Read the model definition and answer for the solid it produces. Units are mm, in the model's axes. Give positions to 0.01 mm unless a question says otherwise; leave off trailing zeros. Write each loop counter-clockwise with the first axis right and the second up, starting at its lowest first coordinate (ties: lowest second). Pieces come first, ordered by that corner, then holes. Notation, with made-up numbers: (31.5, 66) -> (82.5, 66) arc R17 cw to (82.5, 94) -> close; hole circle Ø9 at (-18.75, 28). An arc over 180 degrees is marked (long way). Write item = value, one per line.
from build123d import *

# Parameters (mm, degrees)
SKETCH1_R           = 74.676
BOSS_EXTRUDE1_DEPTH = 3.175
SKETCH2_R           = 7
CUT_EXTRUDE1_DEPTH  = 106.655527906
SKETCH3_R           = 2.25
CUT_EXTRUDE2_DEPTH  = 106.655527906
SKETCH4_R           = 3.175
CUT_EXTRUDE3_DEPTH  = 106.655527906
CUT_EXTRUDE5_REACH  = 107.656
SKETCH6_R           = 6.35


with BuildPart() as part:
    # Sketch1 → Boss-Extrude1 (new body)
    with BuildSketch(Plane(origin=(0, 0, 0), x_dir=(1, 0, 0), z_dir=(0, 1, 0))):
        with Locations(Location((0, 0, 0), (0, 0, 270))):
            Circle(SKETCH1_R)
    extrude(amount=BOSS_EXTRUDE1_DEPTH)

    # Sketch2 → Cut-Extrude1 (cut, through all)
    with BuildSketch(Plane(origin=(0, 3.175, 0), x_dir=(1, 0, 0), z_dir=(0, 1, 0))):
        with Locations(Location((0, 0, 0), (0, 0, 270))):
            Circle(SKETCH2_R)
    extrude(amount=-CUT_EXTRUDE1_DEPTH, mode=Mode.SUBTRACT)

    # Sketch3 → Cut-Extrude2 (cut, through all)
    with BuildSketch(Plane(origin=(0, 3.175, 0), x_dir=(1, 0, 0), z_dir=(0, 1, 0))):
        with Locations(Location((11.314, 0, 0), (0, 0, 270))):
            Circle(SKETCH3_R)
        with Locations(Location((0, -11.314, 0), (0, 0, 270))):
            Circle(SKETCH3_R)
        with Locations(Location((-11.314, 0, 0), (0, 0, 270))):
            Circle(SKETCH3_R)
        with Locations(Location((0, 11.314, 0), (0, 0, 270))):
            Circle(SKETCH3_R)
    extrude(amount=-CUT_EXTRUDE2_DEPTH, mode=Mode.SUBTRACT)

    # Sketch4 → Cut-Extrude3 (cut, through all)
    with BuildSketch(Plane(origin=(0, 3.175, 0), x_dir=(1, 0, 0), z_dir=(0, 1, 0))):
        with Locations(Location((50.8, 0, 0), (0, 0, 270))):
            Circle(SKETCH4_R)
        with Locations(Location((-50.8, 0, 0), (0, 0, 270))):
            Circle(SKETCH4_R)
    extrude(amount=-CUT_EXTRUDE3_DEPTH, mode=Mode.SUBTRACT)

    # Sketch6 → Cut-Extrude5 (cut, up to next)
    with BuildSketch(Plane(origin=(0, 3.175, 0), x_dir=(1, 0, 0), z_dir=(0, 1, 0)), mode=Mode.PRIVATE) as cut_extrude5_sk1:
        with Locations(Location((0, 41.73382544, 0), (0, 0, 270))):
            Circle(SKETCH6_R)
    cut_extrude5_tool1 = extrude(cut_extrude5_sk1.sketch, amount=-CUT_EXTRUDE5_REACH, mode=Mode.PRIVATE) & part.part
    add(cut_extrude5_tool1.solids().sort_by_distance((0, 3.175, -41.733825))[0], mode=Mode.SUBTRACT)


solid = part.part
(1) Given P1, Ø1.5, axis at y = 0.5, z = 35, coming from the -X side; P2, Ø1, axis at y = 2.5, z = -46.5, coming from the -X side, each flat-ended and moving along its own axis, determine where each tip first touches the part or whether it passes through.
Checks:
P1 = -66.36
P2 = -58.83
(2) For a pull along Z with two mould halves and no side action, classify faces 1 (the cylindrical face through (22.431, 1.565, 71.228)), 2 (the cylindrical face through (-6.834, 1.61, -1.517)), 3 (the flat face through (-16, 3.175, -1)) as released by +Z, released by -Z, zero draft, split by the parting line, or undercut.
Checks:
face_1 = split by the parting line
face_2 = undercut
face_3 = zero draft
(3) The part is cut by section B-B on z = -45. Determine the outline of the cut face in (x, y) (1 decimal), plus the area to 3 significant figures.
Checks:
outline = (-59.6, 0) -> (-5.4, 0) -> (-5.4, 3.2) -> (-59.6, 3.2) -> close; (5.4, 0) -> (59.6, 0) -> (59.6, 3.2) -> (5.4, 3.2) -> close
area = 344 mm²
(4) The part is cut by section C-C on x = 50.8. Determine the outline of the cut face in (y, z) (1 decimal), plus the area to 3 significant figures.
Checks:
outline = (0, -54.7) -> (3.2, -54.7) -> (3.2, -3.2) -> (0, -3.2) -> close; (0, 3.2) -> (3.2, 3.2) -> (3.2, 54.7) -> (0, 54.7) -> close
area = 327 mm²
(5) Consider L1, parallel to X at y = 1.75, z = 0 (3 decimals); L2, parallel to Z at x = 10.5, y = 2.55; L3, parallel to Z at x = 49.5, y = 1.55. Determine where each line is inside the solid, lowest interval first.
Checks:
L1 = -74.676 to -53.975, -47.625 to -13.564, -9.064 to -7, 7 to 9.064, 13.564 to 47.625, 53.975 to 74.676
L2 = -73.93 to -2.1, 2.1 to 73.93
L3 = -55.91 to -2.9, 2.9 to 55.91
(6) The part is cut by section A-A on x = 0. Determine the outline of the cut face in (y, z) (3 decimals), plus the area to 3 significant figures.
Checks:
outline = (0, -74.676) -> (3.175, -74.676) -> (3.175, -48.084) -> (0, -48.084) -> close; (0, -35.384) -> (3.175, -35.384) -> (3.175, -13.564) -> (0, -13.564) -> close; (0, -9.064) -> (3.175, -9.064) -> (3.175, -7) -> (0, -7) -> close; (0, 7) -> (3.175, 7) -> (3.175, 9.064) -> (0, 9.064) -> close; (0, 13.564) -> (3.175, 13.564) -> (3.175, 74.676) -> (0, 74.676) -> close
area = 361 mm²
(7) The part is cut by section D-D on y = 2.2. Count the separate pieces of the cut face and the enclosed holes in it, plus the area to 3 significant figures.
Checks:
separate_pieces = 1
enclosed_holes = 8
area = 17,100 mm²
